The listing builds one solid part. Answer for the finished solid, in the listing's coordinates (mm). A direction names the side the tool comes from. Give positions to 0.01 mm unless a question says otherwise; leave off trailing zeros. Order: outer loops, then holes, each group sorted by start corner. A loop starts at its lowest first (then second) coordinate and runs counter-clockwise, first axis right, second up. Notation, with made-up numbers: (-16, -1.75) - (36, -1.75) arc R17 cw to (36, 7.25) - close; hole circle Ø11 at (3.5, 16). An arc over 180 degrees is marked (long way). Use CSV: the item, a comma, the result in double quotes.
```python
from build123d import *

# Parameters (mm, degrees)
F0_W           = 100
F0_H           = 105
F0_W_2         = 40
F0_H_2         = 25
F1_DEPTH       = 3
F2_D           = 3.3
F2_CSINK_D     = 6.72
F2_CSINK_ANGLE = 90
F3_D           = 4.4


with BuildPart() as f1:
    # F0 (on Top) → F1 (new body)
    with BuildSketch(Plane.XY):
        Rectangle(F0_W, F0_H)
        with Locations((0, -15)):
            Rectangle(F0_W_2, F0_H_2, mode=Mode.SUBTRACT)
    extrude(amount=F1_DEPTH)

    # F2 (through all)
    with Locations(Plane(origin=(0, 0, 0), x_dir=(1, 0, 0), z_dir=(0, 0, -1))):
        with Locations((-35, -32.5), (-25, -32.5), (-25, -47.5), (-35, -47.5), (25, -47.5), (25, -32.5), (35, -32.5), (35, -47.5), (25, 32.5), (35, 32.5), (35, 47.5), (25, 47.5), (-25, 47.5), (-35, 47.5), (-35, 32.5), (-25, 32.5)):
            CounterSinkHole(F2_D / 2, F2_CSINK_D / 2, counter_sink_angle=F2_CSINK_ANGLE)

    # F3 (through all)
    with Locations(Plane(origin=(0, 0, 0), x_dir=(1, 0, 0), z_dir=(0, 0, -1))):
        with Locations((27, -5), (27, -20), (-27, -5), (-27, -20)):
            Hole(F3_D / 2)


solid = f1.part
```
Item 1: The part is cut by section A-A (y = -4). Give the vertices of the cut face in (x, z).
Taken from the geometry:
outline,"(-50, 0) - (-20, 0) - (-20, 3) - (-50, 3) - close; (20, 0) - (50, 0) - (50, 3) - (20, 3) - close"
Item 2: Which of the six approach directions +Z, -Z, +X, -X, +Y, -Y give full straight-line access (tool end or side, diameter ignored) to faces 1 (the face through (50, -1, 1)), 2 (the face through (20, -15, 1))?
Taken from the geometry:
face 1,"+Z, -Z, +X, +Y, -Y"
face 2,"+Z, -Z"
Item 3: Each of these flat-tipped pins is pushed along its axis until it touches: pin 1 (3 mm diameter, centred on x = -35, y = 32.5, fed in from -Z); pin 2 (4 mm diameter, centred on x = 25, y = -32.5, fed in from -Z). Where does it stop, or does it pass through?
Taken from the geometry:
pin 1,"through"
pin 2,"z = 1.36"
Item 4: The part is cut by section C-C (y = 32.5). Give the vertices of the cut face in (x, z), and give its area (3 significant figures).
Taken from the geometry:
outline,"(-50, 0) - (-38.36, 0) - (-36.65, 1.71) - (-36.65, 3) - (-50, 3) - close; (-33.35, 1.71) - (-31.64, 0) - (-28.36, 0) - (-26.65, 1.71) - (-26.65, 3) - (-33.35, 3) - close; (-23.35, 1.71) - (-21.64, 0) - (21.64, 0) - (23.35, 1.71) - (23.35, 3) - (-23.35, 3) - close; (26.65, 1.71) - (28.36, 0) - (31.64, 0) - (33.35, 1.71) - (33.35, 3) - (26.65, 3) - close; (36.65, 1.71) - (38.36, 0) - (50, 0) - (50, 3) - (36.65, 3) - close"
area,"249 mm^2"
Item 5: Find the intervals of material crossed by line 1 along X through (y, z) = (-32.5, 2.25); line 2 along Y through (x, z) = (35, 2.55); line 3 along X through (y, z) = (-9.5, 1.15), in increasing order.
Taken from the geometry:
line 1,"-50 to -36.65, -33.35 to -26.65, -23.35 to 23.35, 26.65 to 33.35, 36.65 to 50"
line 2,"-52.5 to -49.15, -45.85 to -34.15, -30.85 to 30.85, 34.15 to 45.85, 49.15 to 52.5"
line 3,"-50 to -20, 20 to 50"
Item 6: The part is cut by section D-D (z = 0.55). Count the separate pieces of the cut face and the enclosed holes in it, and give its area (3 significant figures).
Taken from the geometry:
separate pieces,"1"
enclosed holes,"21"
area,"9,040 mm^2"
Item 7: The part is cut by section B-B (x = -35). Give the vertices of the cut face in (y, z).
Taken from the geometry:
outline,"(-52.5, 0) - (-50.86, 0) - (-49.15, 1.71) - (-49.15, 3) - (-52.5, 3) - close; (-45.85, 1.71) - (-44.14, 0) - (-35.86, 0) - (-34.15, 1.71) - (-34.15, 3) - (-45.85, 3) - close; (-30.85, 1.71) - (-29.14, 0) - (29.14, 0) - (30.85, 1.71) - (30.85, 3) - (-30.85, 3) - close; (34.15, 1.71) - (35.86, 0) - (44.14, 0) - (45.85, 1.71) - (45.85, 3) - (34.15, 3) - close; (49.15, 1.71) - (50.86, 0) - (52.5, 0) - (52.5, 3) - (49.15, 3) - close"
